Job drawing, mm, ordinate dimensions from the low corner. One solid piece. A direction names the side the tool comes from. Give positions to 0.01 mm unless a question says otherwise; leave off trailing zeros. Order: outer loops, then holes, each group sorted by start corner. A loop starts at its lowest first (then second) coordinate and runs counter-clockwise, first axis right, second up. Notation, with made-up numbers: (47.25, 55) - (88.25, 55) arc R21 ccw to (88.25, 83) - close; hole circle Ø2 at (-13, 80.25). An arc over 180 degrees is marked (long way). Use one line per item in the form item = value. Start each with the question number.
1. Tool access for the marked faces 1 and 2: list every direction of +Z, -Z, +X, -X, +Y, -Y with a clear straight run to the whole face (end or side of a thin tool).
2. Band-saw the part on A-A, the plane x = 35. List the corners of the cut face in (y, z).
3. Pin check, flat tips, straight feed: P1, Ø1.5, axis at x = 8.5, z = 3.5, coming from the -Y side; P2, Ø2.5, axis at x = 12, z = 3, coming from the +Y side; P3, Ø1.5, axis at y = 97.5, z = 1.5, coming from the +X side; P4, Ø4, axis at x = 34.5, y = 14, coming from the -Z side. Stop position of each tip, or through.
4. Band-saw the part on C-C, the plane z = 2.9. List the corners of the cut face in (x, y), plus the area to 3 significant figures.
5. Pull direction Y, two halves, no side cores. Call the marked faces 3, 4 and 5: +Y half, -Y half, draft (parallel to the pull), parting line (faces both ways), or undercut.
6. Band-saw the part on B-B, the plane y = 117. List the corners of the cut face in (x, z), plus the area to 3 significant figures.
7. Band-saw the part on D-D, the plane x = 65. List the corners of the cut face in (y, z), plus the area to 3 significant figures.
8. Drill centre lines: line 1 (Y direction, x = 35, z = 1.4); line 2 (Y direction, x = 5, z = 1.2); line 3 (X direction, y = 28.5, z = 4.15). Where is each one in solid material? Low to high.
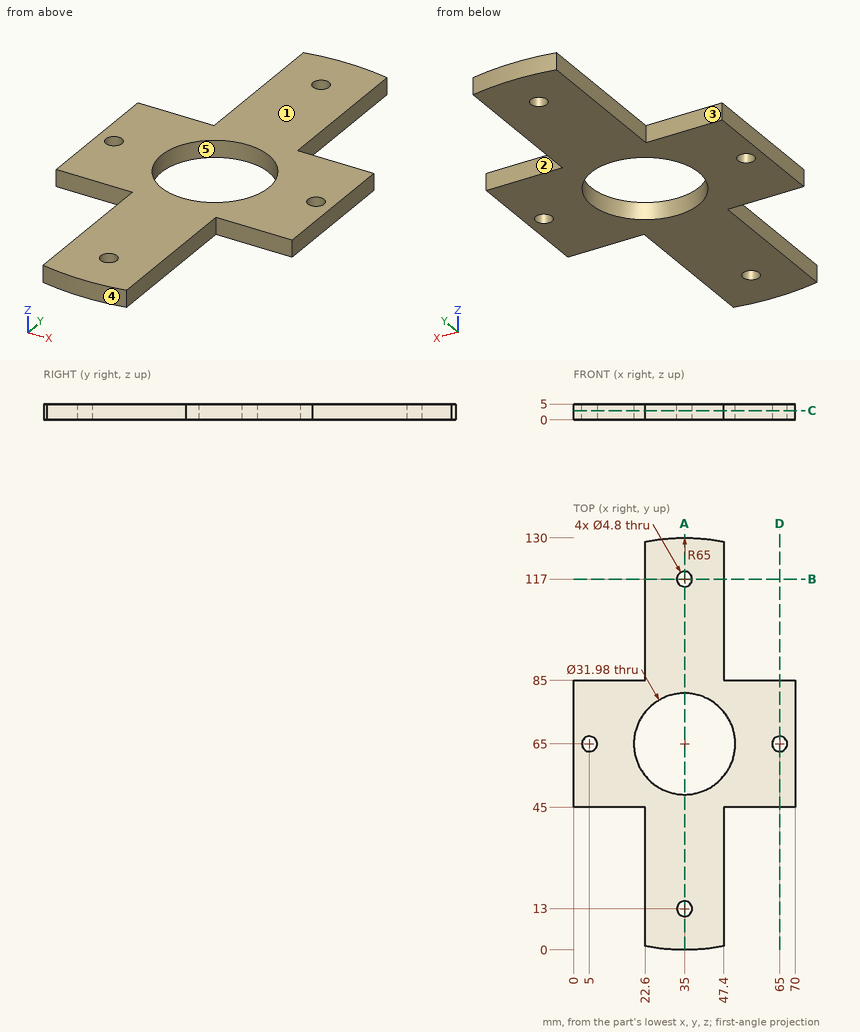
From the geometry:
q1.face_1 = +Z, +X, -X, +Y, -Y
q1.face_2 = +Z, -Z, +X, +Y
q2.outline = (0, 0) - (10.6, 0) - (10.6, 5) - (0, 5) - close; (15.4, 0) - (49.01, 0) - (49.01, 5) - (15.4, 5) - close; (80.99, 0) - (114.6, 0) - (114.6, 5) - (80.99, 5) - close; (119.4, 0) - (130, 0) - (130, 5) - (119.4, 5) - close
q3.P1 = 45
q3.P2 = 85
q3.P3 = 47.4
q3.P4 = 0
q4.outline = (0, 45) - (22.6, 45) - (22.6, 1.19) arc R65 ccw to (47.4, 1.19) - (47.4, 45) - (70, 45) - (70, 85) - (47.4, 85) - (47.4, 128.81) arc R65 ccw to (22.6, 128.81) - (22.6, 85) - (0, 85) - close; hole circle Ø4.8 at (5, 65); hole circle Ø31.98 at (35, 65); hole circle Ø4.8 at (35, 13); hole circle Ø4.8 at (35, 117); hole circle Ø4.8 at (65, 65)
q4.area = 4,140 mm²
q5.face_3 = +Y half
q5.face_4 = -Y half
q5.face_5 = undercut
q6.outline = (22.6, 0) - (32.6, 0) - (32.6, 5) - (22.6, 5) - close; (37.4, 0) - (47.4, 0) - (47.4, 5) - (37.4, 5) - close
q6.area = 100 mm²
q7.outline = (45, 0) - (62.6, 0) - (62.6, 5) - (45, 5) - close; (67.4, 0) - (85, 0) - (85, 5) - (67.4, 5) - close
q7.area = 176 mm²
q8.line_1 = 0 to 10.6, 15.4 to 49.01, 80.99 to 114.6, 119.4 to 130
q8.line_2 = 45 to 62.6, 67.4 to 85
q8.line_3 = 22.6 to 47.4
